Source: CAD feature listing. Evaluate the final solid. Frame: model axes, mm. A direction names the side the tool comes from. Give positions to 0.01 mm unless a question says otherwise; leave off trailing zeros. Order: outer loops, then holes, each group sorted by start corner. A loop starts at its lowest first (then second) coordinate and runs counter-clockwise, first axis right, second up. Notation, with made-up numbers: M 72,40 L 76,40 A20 cw 76,69 Z; hole C -17,16 d4. An arc over 180 degrees is marked long. Use CSV: the item, a comma, the result in double quotes. Start each with the question number.
Item 1: First-contact query: pin 1 (4 mm diameter, centred on x = 88, z = -13.5, fed in from -Y); pin 2 (5 mm diameter, centred on x = -34, y = 115, fed in from -Z); pin 3 (2 mm diameter, centred on y = 111.5, z = -22, fed in from +X). Flat tips, straight axial feed; report the tip coordinate or a pass-through.
Item 2: Section query C-C on y = 57. Return loops of the section in (x, z).
Item 3: Section query B-B on z = 0. Return loops of the section in (x, y), and give its area (3 significant figures).
Item 4: Section query A-A on x = 0. Return loops of the section in (y, z).
Item 5: Pull-direction query (X, two-part tool) for faces 1 (the face through (-1, 130, -9)), 2 (the face through (-44.429, 28.252, -107.155)), 3 (the face through (-15.02, 86.98, -47.69)); classes: +X half, -X half, draft (parallel to the pull), parting line (faces both ways), or undercut.
Item 6: Access query for faces 4 (the face through (-1, 126, -9)), 5 (the face through (2, 50, -52)), 6 (the face through (-4.88, 128.03, -1.08)). Directions: +Z, -Z, +X, -X, +Y, -Y. A direction counts if a zero-diameter tool reaches every point of the face in a straight line with its end or side. Return the directions, or none.
Item 7: Section query D-D on z = 86.5. Return loops of the section in (x, y), and give its area (3 significant figures).
Item 8: Ray query, probe 1 along X at (y, z) = (18, 0); probe 2 along Y at (x, z) = (-21.5, 4.5); probe 3 along Y at (x, z) = (41, -51). Return the intervals inside material, ascending. Write a range as from..to.
from build123d import *

# Parameters (mm, degrees)
BOSS_EXTRUDE1_DEPTH = 100
SKETCH3_R           = 50
BOSS_EXTRUDE3_DEPTH = 80
CHAMFER1_SIZE       = 5
FILLET1_R           = 1
SKETCH4_R           = 5
CUT_EXTRUDE1_DEPTH  = 20
SKETCH5_R           = 15
SKETCH5_R_2         = 2.5
SKETCH5_W           = 60
SKETCH5_H           = 10
SKETCH5_W_2         = 50
CUT_EXTRUDE2_DEPTH  = 20
SKETCH6_W           = 150
SKETCH6_H           = 200
CUT_EXTRUDE3_DEPTH  = 181
SKETCH7_R           = 120
BOSS_EXTRUDE4_DEPTH = 40
SHELL1_T            = -4
SKETCH10_R          = 5
CUT_EXTRUDE4_DEPTH  = 209


with BuildPart() as part:
    # Sketch2 → Boss-Extrude1 (new, symmetric)
    with BuildSketch(Plane.XY):
        with BuildLine():
            Line((-75, 50), (-70, 50))
            ThreePointArc((-70, 50), (-65, 45), (-60, 50))
            Line((-60, 50), (-35, 50))
            Line((-35, 50), (-25, 50))
            Line((-25, 50), (25, 50))
            Line((25, 50), (35, 50))
            Line((35, 50), (60, 50))
            ThreePointArc((60, 50), (65, 45), (70, 50))
            Line((70, 50), (75, 50))
            Line((75, 50), (75, 15))
            ThreePointArc((75, 15), (70.980762114, 0), (75, -15))
            Line((75, -15), (75, -50))
            Line((75, -50), (70, -50))
            ThreePointArc((70, -50), (65, -45), (60, -50))
            Line((60, -50), (35, -50))
            ThreePointArc((35, -50), (30, -45), (25, -50))
            Line((25, -50), (-25, -50))
            ThreePointArc((-25, -50), (-30, -45), (-35, -50))
            Line((-35, -50), (-60, -50))
            ThreePointArc((-60, -50), (-65, -45), (-70, -50))
            Line((-70, -50), (-75, -50))
            Line((-75, -50), (-75, -15))
            ThreePointArc((-75, -15), (-70.980762114, 0), (-75, 15))
            Line((-75, 15), (-75, 50))
        make_face()
    extrude(amount=BOSS_EXTRUDE1_DEPTH, both=True)

    # Sketch3 → Boss-Extrude3 (add)
    with BuildSketch(Plane(origin=(0, 50, 0), x_dir=(1, 0, 0), z_dir=(0, 1, 0))):
        with Locations(Location((0, 0, 0), (0, 0, 90))):
            Circle(SKETCH3_R)
    extrude(amount=BOSS_EXTRUDE3_DEPTH)

    # Chamfer1
    chamfer1_edges = [part.edges().sort_by_distance(p)[0] for p in [
        (0, 130, 50),
    ]]
    chamfer(chamfer1_edges, length=CHAMFER1_SIZE)

    # Fillet1
    fillet1_edges = [part.edges().sort_by_distance(p)[0] for p in [
        (-75, -50, 0),
        (-75, 50, 0),
        (75, 50, 0),
        (75, -50, 0),
    ]]
    fillet(fillet1_edges, radius=FILLET1_R)

    # Sketch4 → Cut-Extrude1 (cut)
    with BuildSketch(Plane.XZ.offset(50)):
        with Locations(Location((-47.5, 80, 0), (0, 0, 270))):
            Circle(SKETCH4_R)
        with Locations(Location((47.5, 80, 0), (0, 0, 270))):
            Circle(SKETCH4_R)
        with Locations(Location((47.5, 40, 0), (0, 0, 270))):
            Circle(SKETCH4_R)
        with Locations(Location((47.5, 0, 0), (0, 0, 270))):
            Circle(SKETCH4_R)
        with Locations(Location((47.5, -40, 0), (0, 0, 270))):
            Circle(SKETCH4_R)
        with Locations(Location((47.5, -80, 0), (0, 0, 270))):
            Circle(SKETCH4_R)
        with Locations(Location((-47.5, 40, 0), (0, 0, 270))):
            Circle(SKETCH4_R)
        with Locations(Location((-47.5, 0, 0), (0, 0, 270))):
            Circle(SKETCH4_R)
        with Locations(Location((-47.5, -40, 0), (0, 0, 270))):
            Circle(SKETCH4_R)
        with Locations(Location((-47.5, -80, 0), (0, 0, 270))):
            Circle(SKETCH4_R)
    extrude(amount=-CUT_EXTRUDE1_DEPTH, mode=Mode.SUBTRACT)

    # Sketch5 → Cut-Extrude2 (cut)
    with BuildSketch(Plane(origin=(0, 0, -100), x_dir=(-1, 0, 0), z_dir=(0, 0, -1))):
        with Locations((40, 25)):
            Circle(SKETCH5_R)
        with Locations((35, 25)):
            Circle(SKETCH5_R_2, mode=Mode.SUBTRACT)
        with Locations((45, 25)):
            Circle(SKETCH5_R_2, mode=Mode.SUBTRACT)
        with Locations((-25, -20)):
            Rectangle(SKETCH5_W, SKETCH5_H)
        with Locations((-25, 10)):
            Rectangle(SKETCH5_W_2, SKETCH5_H)
    extrude(amount=-CUT_EXTRUDE2_DEPTH, mode=Mode.SUBTRACT)

    # Sketch6 → Cut-Extrude3 (cut)
    with BuildSketch(Plane(origin=(0, 50, 0), x_dir=(1, 0, 0), z_dir=(0, 1, 0))):
        Rectangle(SKETCH6_W, SKETCH6_H)
    extrude(amount=-CUT_EXTRUDE3_DEPTH, mode=Mode.SUBTRACT)

    # Sketch7 → Boss-Extrude4 (add)
    with BuildSketch(Plane.XZ.offset(-50)):
        with Locations(Location((0, 0, 0), (0, 0, 270))):
            Circle(SKETCH7_R)
    extrude(amount=BOSS_EXTRUDE4_DEPTH)

    # Shell1
    shell1_openings = [part.faces().sort_by_distance(p)[0] for p in [
        (0, 10, 0),
    ]]
    offset(amount=SHELL1_T, openings=shell1_openings, kind=Kind.INTERSECTION)

    # Sketch10 → Cut-Extrude4 (cut)
    with BuildSketch(Plane(origin=(0, 130, 0), x_dir=(1, 0, 0), z_dir=(0, 1, 0))):
        with Locations(Location((0, 0, 0), (0, 0, 270))):
            Circle(SKETCH10_R)
    extrude(amount=-CUT_EXTRUDE4_DEPTH, mode=Mode.SUBTRACT)


solid = part.part
Verdict:
1,pin 1,"y = 46"
1,pin 2,"z = -38.83"
1,pin 3,"x = 45.38"
2,outline,"C 0,0 d100; hole C 0,0 d92"
3,outline,"M -120,10 L -116,10 L -116,46 L -46,46 L -46,123.34 L -43.34,126 L -5,126 L -5,130 L -45,130 L -50,125 L -50,50 L -120,50 Z; M 5,126 L 43.34,126 L 46,123.34 L 46,46 L 116,46 L 116,10 L 120,10 L 120,50 L 50,50 L 50,125 L 45,130 L 5,130 Z"
3,area,"1,830 mm2"
4,outline,"M 10,-120 L 50,-120 L 50,-50 L 125,-50 L 130,-45 L 130,-5 L 126,-5 L 126,-43.34 L 123.34,-46 L 46,-46 L 46,-116 L 10,-116 Z; M 10,116 L 46,116 L 46,46 L 123.34,46 L 126,43.34 L 126,5 L 130,5 L 130,45 L 125,50 L 50,50 L 50,120 L 10,120 Z"
5,face 1,"draft"
5,face 2,"undercut"
5,face 3,"parting line"
6,face 4,"-Y"
6,face 5,"+Y"
6,face 6,"+Y, -Y"
7,outline,"M -83.17,10 L -77.29,10 L -77.29,46 L 77.29,46 L 77.29,10 L 83.17,10 L 83.17,50 L -83.17,50 Z"
7,area,"1,090 mm2"
8,probe 1,"-120..-116, 116..120"
8,probe 2,"126..130"
8,probe 3,"46..50"
